Autodesk Inventor part; units mm, degrees
ref_plane "YZ Plane" through (0, 0, 0) normal (1, 0, 0) x (0, 1, 0)
ref_plane "XZ Plane" through (0, 0, 0) normal (0, 1, 0) x (-1, 0, 0)
ref_plane "XY Plane" through (0, 0, 0) normal (0, 0, 1) x (1, 0, 0)
ref_plane "Arbeitsebene1" through (0, 0, 0) normal (0, 0, 1) x (1, 0, 0)
sketch "Skizze1" plane through (0, 0, 0) normal (0, 0, 1) x (1, 0, 0)
  circle A0 centre (12, 2.9) radius 1.5
  circle A1 centre (-12, 2.9) radius 1.5
  line L0 (2.5, 12.9) -> (2.5, -7.1)
  line L1 (2.5, -7.1) -> (2.25, -7.1)
  line L2 (2.25, -7.1) -> (2, -7.1)
  line L3 (2, -7.1) -> (1.75, -7.1)
  line L4 (1.75, -7.1) -> (1.5, -7.1)
  line L5 (1.5, -7.1) -> (1.25, -7.1)
  line L6 (1.25, -7.1) -> (1, -7.1)
  line L7 (1, -7.1) -> (0.75, -7.1)
  line L8 (0.75, -7.1) -> (0.5, -7.1)
  line L9 (0.5, -7.1) -> (0.25, -7.1)
  line L10 (0.25, -7.1) -> (0, -7.1)
  line L11 (0, -7.1) -> (-0.25, -7.1)
  line L12 (-0.25, -7.1) -> (-0.5, -7.1)
  line L13 (-0.5, -7.1) -> (-0.75, -7.1)
  line L14 (-0.75, -7.1) -> (-1, -7.1)
  line L15 (-1, -7.1) -> (-1.25, -7.1)
  line L16 (-1.25, -7.1) -> (-1.5, -7.1)
  line L17 (-1.5, -7.1) -> (-1.75, -7.1)
  line L18 (-1.75, -7.1) -> (-2, -7.1)
  line L19 (-2, -7.1) -> (-2.25, -7.1)
  line L20 (-2.25, -7.1) -> (-2.5, -7.1)
  line L21 (-2.5, -7.1) -> (-2.5, 12.9)
  line L22 (-2.5, 12.9) -> (-38, 12.9)
  line L23 (-38, 12.9) -> (-38, -12.9)
  line L24 (-38, -12.9) -> (38, -12.9)
  line L25 (38, -12.9) -> (38, 12.9)
  line L26 (38, 12.9) -> (2.5, 12.9)
  line L27 (35, 11) -> (-35, 11)
  line L28 (-35, 11) -> (-35, -11)
  line L29 (-35, -11) -> (35, -11)
  line L30 (35, -11) -> (35, 11)
  line L31 (35, 11) -> (-35, -11) construction
  line L32 (-35, 11) -> (35, -11) construction
  line L33 (-32.5, 8.5) -> (32.5, 8.5)
  line L34 (32.5, 8.5) -> (32.5, -8.5)
  line L35 (32.5, -8.5) -> (-32.5, -8.5)
  line L36 (-32.5, -8.5) -> (-32.5, 8.5)
  line L37 (-32.5, -8.5) -> (-18.5, -8.5)
  line L38 (-18.5, -8.5) -> (-18.5, 8.5)
  line L39 (-18.5, 8.5) -> (-32.5, 8.5)
  line L40 (-32.5, 8.5) -> (-32.5, -8.5)
  line L41 (32.5, 8.5) -> (18.5, 8.5)
  line L42 (18.5, 8.5) -> (18.5, -8.5)
  line L43 (18.5, -8.5) -> (32.5, -8.5)
  line L44 (32.5, -8.5) -> (32.5, 8.5)
  point P0 (0, 0)
  dimension "d0" = 70
  dimension "d1" = 22
  dimension "d2" = 2.5
  dimension "d5" = 14
  dimension "d6" = 14
extrude "Extrusion1" add sketch "Skizze1" along normal blind 0.5 contours L27 L30 L29 L28 L21 L33 L36 L35 L34 L0 | L0 L33 L21 L27 | L33 L34 L35 L42 | L38 L35 L36 L33
sketch "Skizze2" plane through (0, 0, 0.5) normal (0, 0, 1) x (1, 0, 0)
  circle A0 centre (-29, -0.15) radius 1.6
  circle A1 centre (29, -0.15) radius 1.6
  point P0 (0, 0)
hole "Bohrung1" at (-29, -0.15, 0.5) at (29, -0.15, 0.5) direction (0, 0, -1) diameter 3.5 end through all counterbore diameter 6.5 counterbore depth 2
properties part number "00_Gasket"
Input: part model. Units: mm. Frame: model coordinates. Round coordinates to 2 decimals unless told otherwise and drop trailing zeros. Write each loop counter-clockwise with the first axis right and the second up, starting at its lowest first coordinate (ties: lowest second). Pieces come first, ordered by that corner, then holes.
1) Cut plane D-D (z = 0.3). Return the cut outline in (x, y), then the cut area to 3 significant figures.
2) Ray query, L1, parallel to X at y = -0.15, z = 0.1; L2, parallel to X at y = 6.75, z = 0.45; L3, parallel to Y at x = 29, z = 0.2. Return the intervals inside material, ascending.
3) Cut plane B-B (x = -29). Return the cut outline in (y, z), then the cut area to 3 significant figures.
4) Contact query for a flat-ended pin moving along its axis: P1, Ø5, axis at x = -17, y = -5.5, coming from the -Z side. Output: stop coordinate, or through.
5) Cut plane A-A (y = -7.5). Return the cut outline in (x, z), then the cut area to 3 significant figures.
6) Cut plane C-C (y = -0.15). Return the cut outline in (x, z).
7) Draft query along X for faces 1 (the cylindrical face through (32.173, 0.555, 0.246)), 2 (the cylindrical face through (-25.827, 0.555, 0.246)), 3 (the flat face through (0, -10, 0)). Return one class per face: pulls with the +X half, pulls with the -X half, needs draft (parallel to the pull), parting line crosses it, or undercut.
Geometry says:
1. outline: (-35, -11) - (35, -11) - (35, 11) - (-35, 11) - close; hole circle Ø6.5 at (-29, -0.15); hole (-18.5, -8.5) - (18.5, -8.5) - (18.5, 8.5) - (-18.5, 8.5) - close; hole circle Ø6.5 at (29, -0.15)
1. area: 845 mm2
2. L1: x = -35 to -32.25, -25.75 to -18.5, 18.5 to 25.75, 32.25 to 35
2. L2: x = -35 to -18.5, 18.5 to 35
2. L3: y = -11 to -3.4, 3.1 to 11
3. outline: (-11, 0) - (-3.4, 0) - (-3.4, 0.5) - (-11, 0.5) - close; (3.1, 0) - (11, 0) - (11, 0.5) - (3.1, 0.5) - close
3. area: 7.75 mm2
4. P1: stops at z = 0
5. outline: (-35, 0) - (-18.5, 0) - (-18.5, 0.5) - (-35, 0.5) - close; (18.5, 0) - (35, 0) - (35, 0.5) - (18.5, 0.5) - close
5. area: 16.5 mm2
6. outline: (-35, 0) - (-32.25, 0) - (-32.25, 0.5) - (-35, 0.5) - close; (-25.75, 0) - (-18.5, 0) - (-18.5, 0.5) - (-25.75, 0.5) - close; (18.5, 0) - (25.75, 0) - (25.75, 0.5) - (18.5, 0.5) - close; (32.25, 0) - (35, 0) - (35, 0.5) - (32.25, 0.5) - close
7. face 1: undercut
7. face 2: undercut
7. face 3: needs draft
